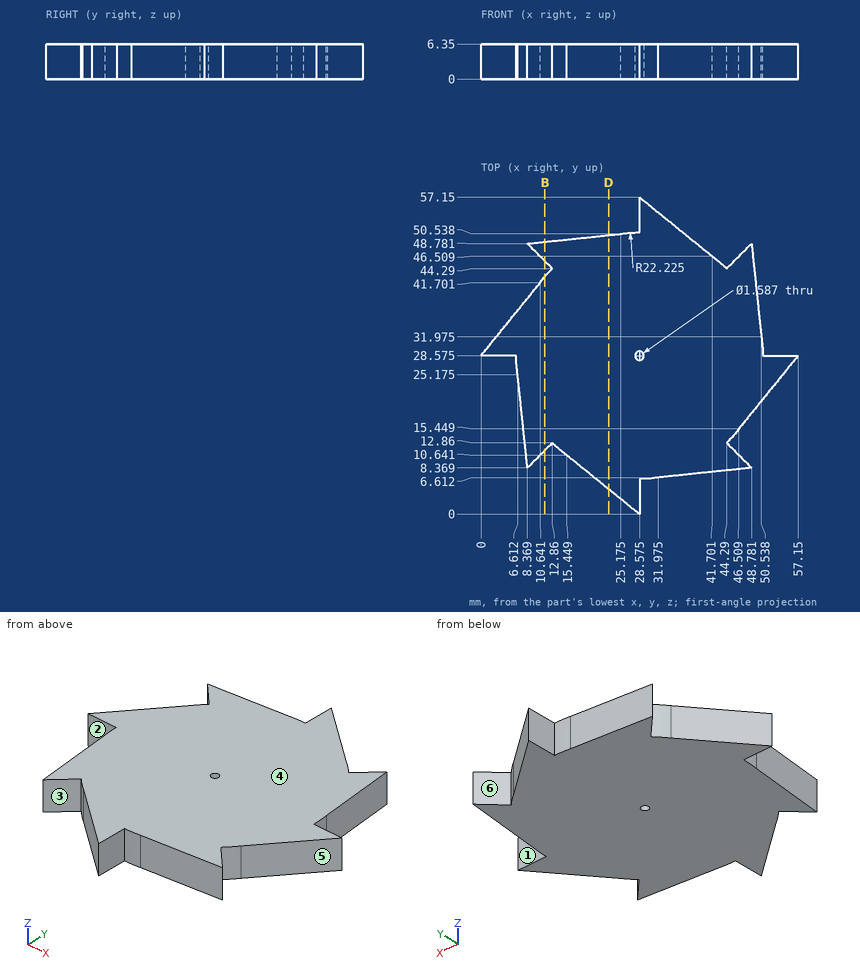
Geometry check sheet. Reference: drawing and pictorial views, mm from the part's lowest x, y, z. A direction names the side the tool comes from. Round coordinates to 2 decimals unless told otherwise and drop trailing zeros. Loops run counter-clockwise (first coordinate to the right, second up) from the corner with the lowest first, then second, coordinate; pieces in that order, holes last. Notation, with made-up numbers: (70, 80.5) - (74, 80.5) arc R3 ccw to (74, 85.5) - close; hole circle Ø6 at (88.25, 85). An arc over 180 degrees is marked (long way). Write item = value, one per line. Start each with the question number.
Q1. Thickness scan on L1, parallel to Y at x = 28, z = 2 (1 decimal); L2, parallel to X at y = 29, z = 4.25 (1 decimal); L3, parallel to X at y = 4, z = 1.25 (1 decimal). Record the ranges inside material, lowest first.
Q2. Section check D-D (x = 23). Record the boundary of the cut face in (y, z), plus the area to 3 significant figures.
Q3. Release check for a two-part mould opening along Y. For the marked faces 4, 5 and 6 record: pulls with the +Y half, pulls with the -Y half, needs draft (parallel to the pull), parting line crosses it, or undercut.
Q4. Section check B-B (x = 11.5). Record the boundary of the cut face in (y, z), plus the area to 3 significant figures.
Q5. Access from +Z, -Z, +X, -X, +Y, -Y to the whole of each face (thin tool, end or side, straight path). Record for the marked faces 1, 2 and 3.
Q6. Depth check by flat-ended pin: P1, Ø3, axis at x = 49, z = 3.5, coming from the +Y side; P2, Ø2, axis at x = 10.5, z = 5.5, coming from the -Y side. Enter the tip coordinate at first touch or a pass-through.
Derived:
q1.L1 = 0.5 to 28, 29.1 to 50.8
q1.L2 = 0.3 to 27.9, 29.2 to 50.8
q1.L3 = 23.6 to 28.6
q2.outline = (4.52, 0) - (50.31, 0) - (50.31, 6.35) - (4.52, 6.35) - close
q2.area = 291 mm^2
q3.face_4 = needs draft
q3.face_5 = undercut
q3.face_6 = pulls with the +Y half
q4.outline = (11.5, 0) - (42.8, 0) - (42.8, 6.35) - (11.5, 6.35) - close; (45.65, 0) - (49.11, 0) - (49.11, 6.35) - (45.65, 6.35) - close
q4.area = 221 mm^2
q5.face_1 = +Z, -Z, +X, +Y
q5.face_2 = +Z, -Z, -X, -Y
q5.face_3 = +Z, -Z, -Y
q6.P1 = 48.78
q6.P2 = 9.5
